Part model, mm, in its own coordinate system. A direction names the side the tool comes from. Round coordinates to 2 decimals unless told otherwise and drop trailing zeros. Order: outer loops, then holes, each group sorted by start corner. A loop starts at its lowest first (then second) coordinate and runs counter-clockwise, first axis right, second up. Notation, with made-up numbers: M 34,84.25 L 88,84.25 A21 ccw 88,89.25 Z; hole C -8.5,25 d8. An arc over 180 degrees is marked long. Write each question's results on one line, items separated by ' | '. Start each with the question number.
1. Band-saw the part on C-C, the plane z = 12.75. List the corners of the cut face in (x, y).
2. Probe L1, parallel to Y at x = 20, z = 1.5; L2, parallel to Z at x = 39.5, y = -2; L3, parallel to X at y = -14, z = 8.75. List the from-to ranges inside material, lowest first. Write a range as [from, to].
3. Band-saw the part on A-A, the plane z = 16. List the corners of the cut face in (x, y).
4. Which spindle directions (+Z, -Z, +X, -X, +Y, -Y) get a long thin tool onto all of the face, cutting with end or side? Do faces 4 (the face through (52.765, -26.348, 8.874)), 5 (the face through (-8.545, 7, 14)), 6 (the face through (7, -7.834, 10)). Say none if no direction does.
5. Drop flat-ended pins along their axis: pin 1 Ø3 at (y, z) = (1.5, 4.5) entering from +X; pin 2 Ø12 at (x, z) = (41.5, 9) entering from -Y; pin 3 Ø5 at (y, z) = (-6.5, 3) entering from -X. Give the stop position or say it passes through.
6. Two-plate mould, pull along Z, no slides. Class faces 1 (the face through (48.072, -17.837, 21.232)), 2 (the face through (22.538, -5.733, 3.877)), 3 (the face through (23, -7, 20)): +Z half, -Z half, draft (parallel to the pull), parting line (faces both ways), or undercut.
7. Band-saw the part on B-B, the plane x = 19. List the corners of the cut face in (y, z), then the cut area to 3 significant figures.
8. Band-saw the part on D-D, the plane y = -27. List the corners of the cut face in (x, z).
```python
from build123d import *

# Parameters (mm, degrees)
PAD003_DEPTH    = 20
POCKET001_DEPTH = 18
SKETCH_W        = 4.5
SKETCH_H        = 8.5
POCKET_DEPTH    = 16.001
PAD_DEPTH       = 18
PAD004_DEPTH    = 3
POCKET002_DEPTH = 12
SKETCH009_R     = 1.5
POCKET003_DEPTH = 33.587329
POCKET004_DEPTH = 10
POCKET005_DEPTH = 4
SKETCH012_R     = 2.95
PAD005_DEPTH    = 2.5


with BuildPart() as part:
    # Sketch004 → Pad003 (new body)
    with BuildSketch(Plane.XY):
        with BuildLine():
            Line((-13.045215, -3.333566), (-13.045215, 3.666434))
            ThreePointArc((-8.545215, 8.166434), (-11.727196, 6.848415), (-13.045215, 3.666434))
            Line((-8.545215, 8.166434), (27.818241, 8.166434))
            ThreePointArc((31.000221, 6.848415), (29.540316, 7.823892), (27.818241, 8.166434))
            Line((31.000221, 6.848415), (56.713067, -18.864432))
            ThreePointArc((56.713067, -25.228393), (58.031087, -22.046412), (56.713067, -18.864432))
            Line((56.713067, -25.228393), (51.76332, -30.17814))
            ThreePointArc((45.399359, -30.17814), (48.581339, -31.49616), (51.76332, -30.17814))
            Line((45.399359, -30.17814), (23.054785, -7.833566))
            Line((23.054785, -7.833566), (-8.545215, -7.833566))
            ThreePointArc((-13.045215, -3.333566), (-11.727196, -6.515546), (-8.545215, -7.833566))
        make_face()
    extrude(amount=PAD003_DEPTH)

    # Sketch005 (on Face12 of Pad003) → Pocket001 (cut)
    with BuildSketch(Plane(origin=(0, 0, 0), x_dir=(1, 0, 0), z_dir=(0, 0, -1))):
        Polygon((-11.045215, -6.166434), (-11.045215, 5.833566), (23.883212, 5.833566), (48.581339, 30.531693), (57.066621, 22.046412), (28.853775, -6.166434), align=None)
    extrude(amount=-POCKET001_DEPTH, mode=Mode.SUBTRACT)

    # Sketch (on Face3 of Pocket001) → Pocket (cut, through all)
    with BuildSketch(Plane.XZ.offset(7.833566)):
        with Locations((-10.795215, 13.75)):
            Rectangle(SKETCH_W, SKETCH_H)
    extrude(amount=-POCKET_DEPTH, mode=Mode.SUBTRACT)

    # Sketch006 (on Face27 of Pocket) → Pad (join)
    with BuildSketch(Plane(origin=(0, 0, 18), x_dir=(1, 0, 0), z_dir=(0, 0, -1))):
        Polygon((21.083212, 5.833566), (21.083212, -6.166434), (28.853775, -6.166434), (34.348392, -0.671817), (25.863111, 7.813465), (23.883212, 5.833566), align=None)
    extrude(amount=PAD_DEPTH)

    # Sketch007 (on Face16 of Pad) → Pad004 (join)
    with BuildSketch(Plane(origin=(0, 0, 0), x_dir=(1, 0, 0), z_dir=(0, 0, -1))):
        Polygon((23.083212, 3.833566), (24.711639, 3.833566), (25.863111, 4.985038), (31.519965, -0.671817), (28.025347, -4.166434), (23.083212, -4.166434), align=None)
    extrude(amount=PAD004_DEPTH)

    # Sketch008 (on Face4 of Pad004) → Pocket002 (cut)
    with BuildSketch(Plane(origin=(0, 0, 0), x_dir=(1, 0, 0), z_dir=(0, 0, -1))):
        with BuildLine():
            Line((21.083212, -6.166434), (21.083212, -8.166434))
            Line((21.083212, -8.166434), (27.818241, -8.166434))
            ThreePointArc((27.818241, -8.166434), (29.540316, -7.823892), (31.000221, -6.848415))
            Line((35.762606, -2.08603), (31.000221, -6.848415))
            Line((34.348392, -0.671817), (35.762606, -2.08603))
            Line((28.853775, -6.166434), (34.348392, -0.671817))
            Line((21.083212, -6.166434), (28.853775, -6.166434))
        make_face()
    extrude(amount=-POCKET002_DEPTH, mode=Mode.SUBTRACT)

    # Sketch009 (on DatumPlane) → Pocket003 (cut, through all)
    with BuildSketch(Plane(origin=(20.996104, -12.803661, 1.052949), x_dir=(-0.003926, -0.009478, -0.999947), z_dir=(0.382663, 0.923831, -0.010259))):
        with Locations((-5.157433, 0)):
            Circle(SKETCH009_R)
    extrude(amount=POCKET003_DEPTH, mode=Mode.SUBTRACT)

    # Sketch010 (on DatumPlane) → Pocket004 (cut)
    with BuildSketch(Plane(origin=(20.996104, -12.803661, 1.052949), x_dir=(-0.003926, -0.009478, -0.999947), z_dir=(0.382663, 0.923831, -0.010259))):
        Polygon((-3.657433, -2.598076), (-2.157433, 0), (-3.657433, 2.598076), (-6.657433, 2.598076), (-8.157433, 0), (-6.657433, -2.598076), align=None)
    extrude(amount=POCKET004_DEPTH, mode=Mode.SUBTRACT)

    # Sketch011 (on Face47 of Pocket004) → Pocket005 (cut)
    with BuildSketch(Plane(origin=(0, 0, 18), x_dir=(1, 0, 0), z_dir=(0, 0, -1))):
        Polygon((21.083212, 5.833566), (21.083212, -6.166434), (28.853775, -6.166434), (34.348392, -0.671817), (25.863111, 7.813465), (23.883212, 5.833566), align=None)
    extrude(amount=POCKET005_DEPTH, mode=Mode.SUBTRACT)

    # Sketch012 (on Face7 of Pocket005) → Pad005 (join)
    with BuildSketch(Plane.XY.offset(20)):
        with Locations((-0.345215, 0)):
            Circle(SKETCH012_R)
        with Locations((45.257938, -18.72301)):
            Circle(SKETCH012_R)
    extrude(amount=PAD005_DEPTH)


solid = part.part
```
Solution:
1) outline: M -8.55,-7.83 L 23.05,-7.83 L 45.4,-30.18 A4.5 ccw 51.76,-30.18 L 56.71,-25.23 A4.5 ccw 56.71,-18.86 L 31,6.85 A4.5 ccw 27.82,8.17 L -8.55,8.17 L -8.55,6.17 L 21.08,6.17 L 21.08,-5.83 L -8.55,-5.83 Z; hole M 25.86,-7.81 L 48.58,-30.53 L 57.07,-22.05 L 34.35,0.67 Z
2) L1: [-7.83, -5.83], [6.17, 8.17] | L2: [0, 20] | L3: [29.22, 32.05], [49.02, 51.85]
3) outline: M -8.55,-7.83 L 23.05,-7.83 L 45.4,-30.18 A4.5 ccw 51.76,-30.18 L 56.71,-25.23 A4.5 ccw 56.71,-18.86 L 31,6.85 A4.5 ccw 27.82,8.17 L -8.55,8.17 L -8.55,6.17 L 28.85,6.17 L 57.07,-22.05 L 48.58,-30.53 L 23.88,-5.83 L -8.55,-5.83 Z
4) face 4: -Z | face 5: -X, +Y, -Y | face 6: +Z, -Z, -X, -Y
5) pin 1: x = 37.85 | pin 2: y = -31.36 | pin 3: x = -13
6) face 1: draft | face 2: undercut | face 3: +Z half
7) outline: M -7.83,0 L -5.83,0 L -5.83,18 L 6.17,18 L 6.17,0 L 8.17,0 L 8.17,20 L -7.83,20 Z | area: 104 mm^2
8) outline: M 42.22,0 L 45.05,0 L 45.05,18 L 52.11,18 L 52.11,0 L 54.94,0 L 54.94,20 L 42.22,20 Z
